Build history of the part. All positions in model axes, mm. Face numbers are marked on the shaded views. A direction names the side the tool comes from. Coordinates: 2 decimals unless noted, no trailing zeros. Loops run counter-clockwise (first coordinate to the right, second up) from the corner with the lowest first, then second, coordinate; pieces in that order, holes last.
Item 1: Cut at B-B (y = -12). List the corners of the cut face in (x, z), and give its area (3 significant figures).
Item 2: Drill centre lines: line 1 along X through (y, z) = (-10, -37); line 2 along Z through (x, y) = (0.5, 5.5); line 3 along Z through (x, y) = (23, -7). Where is each one in solid material? Low to high.
Item 3: 3-axis set-ups, long thin cutter, end or side, ignore diameter. For the marked faces 1, 2 and 3: which of +Z, -Z, +X, -X, +Y, -Y reach the whole face in a straight line?
Item 4: Mould opens along X. For the marked faces 4, 5 and 6 say: released by +X, released by -X, zero draft, split by the parting line, or undercut.
Item 5: Cut at A-A (z = 45). List the corners of the cut face in (x, y), and give its area (3 significant figures).
Item 6: Cut at C-C (y = -7.5). Count the separate pieces of the cut face and the enclosed holes in it, and give its area (3 significant figures).
Item 7: Cut at D-D (y = 15). List the corners of the cut face in (x, z).
Item 8: Flat gauge pins, fed straight in: pin 1 (15 mm diameter, centred on x = 6.5, z = -24.5, fed in from +Y); pin 2 (12 mm diameter, centred on x = 2.5, z = -10, fed in from -Y); pin 3 (10 mm diameter, centred on y = 19.5, z = 50, fed in from -X). Where does each tip first touch, or does it go through?
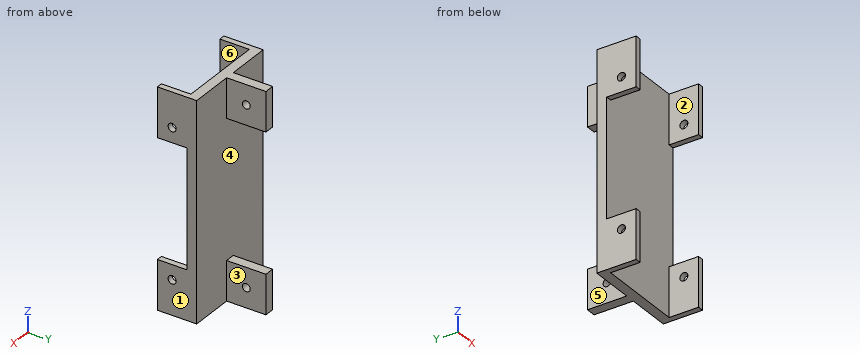
Autodesk Inventor part; units mm, degrees
ref_plane "YZ Plane" through (0, 0, 0) normal (1, 0, 0) x (0, 1, 0)
ref_plane "XZ Plane" through (0, 0, 0) normal (0, 1, 0) x (-1, 0, 0)
ref_plane "XY Plane" through (0, 0, 0) normal (0, 0, 1) x (1, 0, 0)
sketch "Sketch1" plane through (0, 0, 0) normal (0, 1, 0) x (-1, 0, 0)
  line L0 (25, 55) -> (-25, 55)
  line L1 (-25, 55) -> (-25, -55)
  line L2 (-25, -55) -> (25, -55)
  line L3 (25, -55) -> (25, 55)
  line L4 (25, 55) -> (-25, -55) construction
  line L5 (-25, 55) -> (25, -55) construction
  point P0 (0, 0)
  dimension "d0" = 50
  dimension "d1" = 110
extrude "Extrusion1" add sketch "Sketch1" along normal blind 5
sketch "Sketch2" plane through (0, 0, 0) normal (0, -1, 0) x (1, 0, 0)
  line L0 (25, 55) -> (25, -55)
  line L1 (-25, 55) -> (25, 55)
  line L2 (-25, -55) -> (-25, 55)
  line L3 (25, -55) -> (-25, -55)
  line L4 (25, 55) -> (22, 55)
  line L5 (22, 55) -> (22, 30)
  line L6 (22, 30) -> (25, 30)
  line L7 (25, 30) -> (25, 55)
  line L8 (-25, 55) -> (-22, 55)
  line L9 (-22, 55) -> (-22, 30)
  line L10 (-22, 30) -> (-25, 30)
  line L11 (-25, 30) -> (-25, 55)
  line L12 (25, -55) -> (22, -55)
  line L13 (22, -55) -> (22, -30)
  line L14 (22, -30) -> (25, -30)
  line L15 (25, -30) -> (25, -55)
  line L16 (-25, -55) -> (-22, -55)
  line L17 (-22, -55) -> (-22, -30)
  line L18 (-22, -30) -> (-25, -30)
  line L19 (-25, -30) -> (-25, -55)
  point P0 (0, 0)
  dimension "d4" = 3
  dimension "d5" = 3
  dimension "d6" = 3
  dimension "d7" = 25
  dimension "d8" = 25
  dimension "d9" = 25
  dimension "d10" = 25
extrude "Extrusion2" add sketch "Sketch2" along normal blind 15 contours L0 L6 L5 L1 | L0 L3 L13 L14 | L9 L10 L2 L1 | L3 L2 L18 L17
sketch "Sketch3" plane through (25, 5, 55) normal (1, 0, 0) x (0, 0, -1)
  circle A0 centre (17.5, -12.5) radius 2.05
  circle A1 centre (92.5, -12.5) radius 2.05
  line L0 (25, -20) -> (0, -20)
  line L1 (110, -20) -> (85, -20)
  line L2 (85, -5) -> (85, -20)
  line L3 (25, -5) -> (25, -20)
  point P0 (55, -5)
  dimension "d13" = 4.1
  dimension "d14" = 4.1
  dimension "d15" = 7.5
  dimension "d16" = 7.5
  dimension "d17" = 7.5
  dimension "d18" = 7.5
extrude "Extrusion3" cut sketch "Sketch3" against normal through all
sketch "Sketch5" plane through (0, 0, 0) normal (1, 0, 0) x (0, 1, 0)
  line L0 (25, 55) -> (5, 55)
  line L1 (5, 55) -> (5, 35)
  line L2 (5, 35) -> (25, 35)
  line L3 (25, 35) -> (25, 55)
  line L4 (25, -35) -> (5, -35)
  line L5 (5, -35) -> (5, -55)
  line L6 (5, -55) -> (25, -55)
  line L7 (25, -55) -> (25, -35)
  line L8 (5, 55) -> (5, -55)
  line L9 (-15, -55) -> (5, -55)
  line L10 (5, 55) -> (-15, 55)
  point P0 (0, 0)
  dimension "d21" = 20
  dimension "d22" = 20
  dimension "d23" = 20
  dimension "d24" = 20
extrude "Extrusion4" add sketch "Sketch5" along normal mid plane 5
sketch "Sketch6" plane through (2.5, 0, 0) normal (1, 0, 0) x (0, 0, -1)
  line L0 (-35, 5) -> (-55, 5)
  line L1 (-35, 5) -> (-35, 25)
  line L2 (-35, 25) -> (-55, 25)
  line L3 (-55, 25) -> (-55, 5)
  line L4 (35, 25) -> (35, 5)
  line L5 (55, 5) -> (35, 5)
  line L6 (55, 5) -> (55, 25)
  line L7 (55, 25) -> (35, 25)
  circle A0 centre (-45, 15) radius 2
  circle A1 centre (45, 15) radius 2
  point P0 (0, 0)
  dimension "d29" = 4
  dimension "d30" = 4
extrude "Extrusion5" cut sketch "Sketch6" against normal blind 5 contours A0 | A1
properties part number "gripper_case_bracket"
Filled sheet:
1. outline: (-25, -55) - (-22, -55) - (-22, -30) - (-25, -30) - close; (-25, 30) - (-22, 30) - (-22, 55) - (-25, 55) - close; (22, -55) - (25, -55) - (25, -30) - (22, -30) - close; (22, 30) - (25, 30) - (25, 55) - (22, 55) - close
1. area: 300 mm2
2. line 1: x = -25 to -22, 22 to 25
2. line 2: z = -55 to -35, 35 to 55
2. line 3: z = -55 to -39.49, -35.51 to -30, 30 to 35.51, 39.49 to 55
3. face 1: +Z, -Z, +X, +Y, -Y
3. face 2: +Z, -Z, -Y
3. face 3: +Z, -Z, +X, +Y
4. face 4: zero draft
4. face 5: released by -X
4. face 6: undercut
5. outline: (-25, -15) - (-22, -15) - (-22, 0) - (22, 0) - (22, -15) - (25, -15) - (25, 5) - (2.5, 5) - (2.5, 13) - (-2.5, 13) - (-2.5, 5) - (-25, 5) - close; (-2.5, 17) - (2.5, 17) - (2.5, 25) - (-2.5, 25) - close
5. area: 420 mm2
6. separate pieces: 8
6. enclosed holes: 0
6. area: 251 mm2
7. outline: (-2.5, -55) - (2.5, -55) - (2.5, -47) - (-2.5, -47) - close; (-2.5, -43) - (2.5, -43) - (2.5, -35) - (-2.5, -35) - close; (-2.5, 35) - (2.5, 35) - (2.5, 43) - (-2.5, 43) - close; (-2.5, 47) - (2.5, 47) - (2.5, 55) - (-2.5, 55) - close
8. pin 1: stops at y = 5
8. pin 2: stops at y = 0
8. pin 3: stops at x = -2.5
